Could you check a few things on this model? Use its own coordinates, in mm. A direction names the side the tool comes from. Coordinates: 2 decimals unless noted, no trailing zeros. Loops run counter-clockwise (first coordinate to the right, second up) from the corner with the lowest first, then second, coordinate; pieces in that order, holes last.
from build123d import *

# Parameters (mm, degrees)
F0_W      = 50
F0_H      = 40
F1_DEPTH  = 25
F2_W      = 48
F2_H      = 38
F3_DEPTH  = 19
F4_W      = 5
F4_H      = 5
F4_W_2    = 4.9955489208
F5_DEPTH  = 19
F6_R      = 1.5
F7_DEPTH  = 10
F8_R      = 2.5
F8_R_2    = 1.5
F9_DEPTH  = 5
F10_DEPTH = 10
F11_R     = 5
F12_DEPTH = 2
F13_R     = 1.5
F14_DEPTH = 5


with BuildPart() as f1:
    # F0 (on Top) → F1 (new body)
    with BuildSketch(Plane.XY):
        with Locations((-24.0044510792, 35.204609856)):
            Rectangle(F0_W, F0_H)
    extrude(amount=F1_DEPTH)

    # F2 (on face) → F3 (cut)
    with BuildSketch(Plane.XY.offset(25)):
        with Locations((-24.0044510792, 35.204609856)):
            Rectangle(F2_W, F2_H)
    extrude(amount=-F3_DEPTH, mode=Mode.SUBTRACT)

    # F4 (on face) → F5 (join)
    with BuildSketch(Plane.XY.offset(6)):
        with Locations((-45.5044510792, 51.704609856)):
            Rectangle(F4_W, F4_H)
        with Locations((-45.5044510792, 18.704609856)):
            Rectangle(F4_W, F4_H)
        with Locations((-2.5022255396, 51.704609856)):
            Rectangle(F4_W_2, F4_H)
        with Locations((-2.5044510792, 18.704609856)):
            Rectangle(F4_W, F4_H)
    extrude(amount=F5_DEPTH)

    # F6 (on face) → F7 (cut)
    with BuildSketch(Plane.XY.offset(25)):
        with Locations((-45.5044510792, 51.704609856)):
            Circle(F6_R)
        with Locations((-45.5044510792, 18.704609856)):
            Circle(F6_R)
        with Locations((-2.5044510792, 18.704609856)):
            Circle(F6_R)
        with Locations((-2.5022255396, 51.704609856)):
            Circle(F6_R)
    extrude(amount=-F7_DEPTH, mode=Mode.SUBTRACT)

    # F8 (on face) → F9 (join)
    with BuildSketch(Plane.XY.offset(6)):
        with Locations((-28.0044510792, 31.204609856)):
            Circle(F8_R)
        with Locations((-28.0044510792, 31.204609856)):
            Circle(F8_R_2, mode=Mode.SUBTRACT)
        with Locations((-13.0044510792, 41.204609856)):
            Circle(F8_R)
        with Locations((-13.0044510792, 41.204609856)):
            Circle(F8_R_2, mode=Mode.SUBTRACT)
    extrude(amount=F9_DEPTH)

    # F10 (cut): faces of the model
    f10_faces = [f1.faces().sort_by_distance(p)[0] for p in [
        (-28.0044510792, 31.204609856, 6),
        (-13.0044510792, 41.204609856, 6),
    ]]
    extrude(f10_faces, amount=-F10_DEPTH, mode=Mode.SUBTRACT)

    # F11 (on face) → F12 (join)
    with BuildSketch(Plane.XY.offset(6)):
        with Locations((-28.0044510792, 31.204609856)):
            Circle(F11_R)
        with Locations((-13.0044510792, 41.204609856)):
            Circle(F11_R)
    extrude(amount=F12_DEPTH)

    # F13 (on face) → F14 (cut)
    with BuildSketch(Plane(origin=(0, 0, 0), x_dir=(1, 0, 0), z_dir=(0, 0, -1))):
        Polygon((-25.0050230309, -31.2631878667), (-26.4540070097, -28.6363179747), (-29.453435058, -28.5777399641), (-31.0038791275, -31.1460318454), (-29.5548951487, -33.7729017373), (-26.5554671004, -33.8314797479), align=None)
        with Locations((-28.0044510792, -31.204609856)):
            Circle(F13_R, mode=Mode.SUBTRACT)
        Polygon((-10.2501344474, -42.3936178003), (-10.5975816782, -39.4138056549), (-13.3518983101, -38.2247977106), (-15.758767711, -40.0156019117), (-15.4113204802, -42.9954140571), (-12.6570038483, -44.1844220014), align=None)
        with Locations((-13.0044510792, -41.204609856)):
            Circle(F13_R, mode=Mode.SUBTRACT)
    extrude(amount=F14_DEPTH, mode=Mode.SUBTRACT)


solid = f1.part
(1) Imagine slicing it at B-B, the plane y = 22.5. Write out the boundary of the cut face in (x, z), and give its area (3 significant figures).
Answers:
outline: (-49, 0) - (1, 0) - (1, 25) - (0, 25) - (0, 6) - (-48, 6) - (-48, 25) - (-49, 25) - close
area: 338 mm2
(2) I need wall thicknesses on probe 1 along X at (y, z) = (31, 6.5); probe 2 along X at (y, z) = (29.5, 18); probe 3 along Y at (x, z) = (-34, 11.5). Which ranges of each line are inside material? Lowest first, please.
Answers:
probe 1: x = -49 to -48, -33 to -23.01, 0 to 1
probe 2: x = -49 to -48, 0 to 1
probe 3: y = 15.2 to 16.2, 54.2 to 55.2
(3) Imagine slicing it at D-D, the plane z = 17.75. Write out the boundary of the cut face in (x, y).
Answers:
outline: (-49, 15.2) - (1, 15.2) - (1, 55.2) - (-49, 55.2) - close; hole (-48, 21.2) - (-43, 21.2) - (-43, 16.2) - (-5, 16.2) - (-5, 21.2) - (0, 21.2) - (0, 49.2) - (-5, 49.2) - (-5, 54.2) - (-43, 54.2) - (-43, 49.2) - (-48, 49.2) - close; hole circle Ø3 at (-45.5, 18.7); hole circle Ø3 at (-45.5, 51.7); hole circle Ø3 at (-2.5, 18.7); hole circle Ø3 at (-2.5, 51.7)
(4) Imagine slicing it at C-C, the plane x = -20. Write out the boundary of the cut face in (y, z), and give its area (3 significant figures).
Answers:
outline: (15.2, 0) - (55.2, 0) - (55.2, 25) - (54.2, 25) - (54.2, 6) - (16.2, 6) - (16.2, 25) - (15.2, 25) - close
area: 278 mm2
(5) We'd pull the mould along Y, two halves only. Please class faces 1 (the face through (-46, 19, 15)), 2 (the face through (-48.2, 35.3, 25)), 3 (the face through (-24, 55.205, 12)), 4 (the face through (-28.2, 32.69, 9.48)): +Y half, -Y half, draft (parallel to the pull), parting line (faces both ways), or undercut.
Answers:
face 1: undercut
face 2: draft
face 3: +Y half
face 4: undercut
(6) Imagine slicing it at A-A, the plane z = 6.75. Write out the boundary of the cut face in (x, y).
Answers:
outline: (-49, 15.2) - (1, 15.2) - (1, 55.2) - (-49, 55.2) - close; circle Ø10 at (-28, 31.2); circle Ø10 at (-13, 41.2); hole (-48, 21.2) - (-43, 21.2) - (-43, 16.2) - (-5, 16.2) - (-5, 21.2) - (0, 21.2) - (0, 49.2) - (-5, 49.2) - (-5, 54.2) - (-43, 54.2) - (-43, 49.2) - (-48, 49.2) - close
(7) Which directions (+Z, -Z, +X, -X, +Y, -Y) give clear straight access to the entire face, cutting with the end or side of a thin tool? Please do faces 5 (the face through (-13.546, 38.764, 9.479)), 6 (the face through (-28.2, 32.69, 3.04)).
Answers:
face 5: +Z
face 6: -Z
(8) For pin 1 (3 mm diameter, centred on x = -30, y = 31.5, fed in from +Z); pin 2 (11.5 mm diameter, centred on x = -24.5, y = 43, fed in from +Z); pin 3 (2.5 mm diameter, centred on x = -28, y = 31.2, fed in from +Z), each with a flat end and sliding along its axis, tell me the tip position at first contact or that it passes through.
Answers:
pin 1: stops at z = 11
pin 2: stops at z = 6
pin 3: stops at z = 8
